```python
from build123d import *

# Parameters (mm, degrees)
SKETCH1_W                = 100
SKETCH1_H                = 100
BOSS_EXTRUDE1_DEPTH      = 50
BOSS_EXTRUDE1_DEPTH_BACK = 50
SKETCH2_R                = 25
BOSS_EXTRUDE2_DEPTH      = 60


with BuildPart() as part:
    # Sketch1 → Boss-Extrude1 (new body, two sides)
    with BuildSketch(Plane.XY) as boss_extrude1_sk:
        Rectangle(SKETCH1_W, SKETCH1_H)
    extrude(amount=BOSS_EXTRUDE1_DEPTH)
    extrude(boss_extrude1_sk.sketch, amount=-BOSS_EXTRUDE1_DEPTH_BACK)

    # Sketch2 → Boss-Extrude2 (add)
    with BuildSketch(Plane.XY.offset(100)):
        Circle(SKETCH2_R)
    extrude(amount=-BOSS_EXTRUDE2_DEPTH)


solid = part.part
```
Check sheet for the modelled part. Datum: model origin and axes. Units: mm. A direction names the side the tool comes from. Coordinates: 2 decimals unless noted, no trailing zeros. Order: outer loops, then holes, each group sorted by start corner. A loop starts at its lowest first (then second) coordinate and runs counter-clockwise, first axis right, second up. Notation, with made-up numbers: (22.5, 35) -> (36.5, 35) arc R16 cw to (36.5, 62) -> close; hole circle Ø11 at (-23, 42.25). An arc over 180 degrees is marked (long way). Write each question's results on one line, items separated by ' | '. Start each with the question number.
1) Material ranges on line 1 along Z through (x, y) = (11, -38); line 2 along Y through (x, z) = (-11.5, 83); line 3 along X through (y, z) = (-20, 94), recorded low to high.
2) Section check B-B (x = 0). Enter the section's corners in (y, z).
3) Depth check by flat-ended pin: pin 1 (3 mm diameter, centred on x = 16, z = 52.5, fed in from +Y); pin 2 (12 mm diameter, centred on x = 2, z = 71, fed in from -Y); pin 3 (3 mm diameter, centred on x = -17.5, z = 83, fed in from -Y). Enter the tip coordinate at first touch or a pass-through.
4) Section check D-D (y = 36). Enter the section's corners in (x, z).
5) Section check C-C (z = 89). Enter the section's corners in (x, y), and give its area (3 significant figures).
6) Set-up check for faces 1 (the face through (-50, -1, 1)), 2 (the face through (23.846, 7.509, 75.35)): record each of +Z, -Z, +X, -X, +Y, -Y from which the full face is reachable in a straight line by a thin tool's end or side.
7) Section check A-A (y = -20). Enter the section's corners in (x, z), and give its area (3 significant figures).
Checked values:
1) line 1: -50 to 50 | line 2: -22.2 to 22.2 | line 3: -15 to 15
2) outline: (-50, -50) -> (50, -50) -> (50, 50) -> (25, 50) -> (25, 100) -> (-25, 100) -> (-25, 50) -> (-50, 50) -> close
3) pin 1: y = 20.37 | pin 2: y = -25 | pin 3: y = -19.21
4) outline: (-50, -50) -> (50, -50) -> (50, 50) -> (-50, 50) -> close
5) outline: circle Ø50 at (0, 0) | area: 1,960 mm²
6) face 1: +Z, -Z, -X, +Y, -Y | face 2: +Z
7) outline: (-50, -50) -> (50, -50) -> (50, 50) -> (15, 50) -> (15, 100) -> (-15, 100) -> (-15, 50) -> (-50, 50) -> close | area: 11,500 mm²
